Read the model definition and answer for the solid it produces. Units are mm, in the model's axes. Coordinates: 2 decimals unless noted, no trailing zeros. Write each loop counter-clockwise with the first axis right and the second up, starting at its lowest first coordinate (ties: lowest second). Pieces come first, ordered by that corner, then holes.
from build123d import *

# Parameters (mm, degrees)
SKETCH1_R               = 38.1
BOSS_EXTRUDE1_DEPTH     = 12.7
FILLET1_R               = 12.7
CUT_EXTRUDE1_DEPTH      = 60.56828015
CUT_EXTRUDE1_DEPTH_BACK = 60.56828015
SKETCH2_R               = 9.999999939


with BuildPart() as part:
    # Sketch1 → Boss-Extrude1 (new, symmetric)
    with BuildSketch(Plane.XY):
        Circle(SKETCH1_R)
    extrude(amount=BOSS_EXTRUDE1_DEPTH, both=True)

    # Fillet1
    fillet1_edges = [part.edges().sort_by_distance(p)[0] for p in [
        (-38.1, 0, -12.7),
        (-38.1, 0, 12.7),
    ]]
    fillet(fillet1_edges, radius=FILLET1_R - 0.0001)  # a hair under: the kernel refuses the full size

    # Sketch2 → Cut-Extrude1 (cut, two sides: drawn at the far end of the back side and taken through both)
    with BuildSketch(Plane.XY.offset(12.7).offset(-CUT_EXTRUDE1_DEPTH_BACK)):
        Circle(SKETCH2_R)
    extrude(amount=CUT_EXTRUDE1_DEPTH + CUT_EXTRUDE1_DEPTH_BACK, mode=Mode.SUBTRACT)


solid = part.part
Item 1: The part is cut by section D-D (z = -3). Give the vertices of the cut face in (x, y).
Item 2: The part is cut by section C-C (z = 5.75). Give the vertices of the cut face in (x, y), and give its area (3 significant figures).
Item 3: Find the intervals of material crossed by probe 1 along Y at (x, z) = (0, -3.75); probe 2 along Y at (x, z) = (0, -4.75); probe 3 along Z at (x, y) = (22, 14), in increasing order.
Item 4: Determine the mould class of faces 1 (the flat face through (11, 0, -12.7)), 2 (the cylindrical face through (4.614, -8.872, -0.178)) for opening direction Y: +Y half, -Y half, draft (parallel to the pull), parting line (faces both ways), or undercut.
Item 5: Given pin 1 (6 mm diameter, centred on x = -7, z = 0, fed in from +Y); pin 2 (1 mm diameter, centred on x = 26.5, z = -5.5, fed in from -Y); pin 3 (3 mm diameter, centred on x = 16, z = 7, fed in from -Y), each flat-ended and moving along its own axis, determine where each tip first touches the part or whether it passes through.
Answer:
1. outline: circle Ø75.48 at (0, 0); hole circle Ø20 at (0, 0)
2. outline: circle Ø73.45 at (0, 0); hole circle Ø20 at (0, 0)
2. area: 3,920 mm2
3. probe 1: y = -37.53 to -10, 10 to 37.53
3. probe 2: y = -37.18 to -10, 10 to 37.18
3. probe 3: z = -12.68 to 12.68
4. face 1: draft
4. face 2: undercut
5. pin 1: stops at y = 37.89
5. pin 2: stops at y = -26.21
5. pin 3: stops at y = -33.45
